Could you check a few things on this model? Use its own coordinates, in mm. Coordinates: 2 decimals unless noted, no trailing zeros. Loops run counter-clockwise (first coordinate to the right, second up) from the corner with the lowest first, then second, coordinate; pieces in that order, holes last. Notation, with made-up numbers: M 62.25,-8.5 L 117.25,-8.5 A22 cw 117.25,7.5 Z; hole C 57.25,-32.75 d1. An arc over 180 degrees is marked long. Write each question's results on one line, items separated by ' | '.
```python
from build123d import *

# Parameters (mm, degrees)
SKETCH2_W           = 31.75
SKETCH2_H           = 22.86
SKETCH2_R           = 3.2766
SKETCH2_H_2         = 12.7
SKETCH2_R_2         = 2.0828
SKETCH2_H_3         = 10.16
BOSS_EXTRUDE1_DEPTH = 1.5875


with BuildPart() as part:
    # Sketch2 → Boss-Extrude1 (new body)
    # profile 1 of 4: a face of its own
    with BuildSketch(Plane.XY):
        with Locations((15.875, 11.43)):
            Rectangle(SKETCH2_W, SKETCH2_H)
        with Locations((15.875, 11.43)):
            Circle(SKETCH2_R, mode=Mode.SUBTRACT)
    # profile 2 of 4: a face of its own
    with BuildSketch(Plane.XY):
        with Locations((15.875, 29.21)):
            Rectangle(SKETCH2_W, SKETCH2_H_2)
        with Locations((9.525, 29.21)):
            Circle(SKETCH2_R_2, mode=Mode.SUBTRACT)
        with Locations((22.225, 29.21)):
            Circle(SKETCH2_R_2, mode=Mode.SUBTRACT)
    # profile 3 of 4: a face of its own
    with BuildSketch(Plane.XY):
        with Locations((15.875, 40.64)):
            Rectangle(SKETCH2_W, SKETCH2_H_3)
    # profile 4 of 4: a face of its own
    with BuildSketch(Plane.XY):
        Polygon((31.75, 53.041010695), (31.75, 45.72), (0, 45.72), align=None)
    extrude(amount=BOSS_EXTRUDE1_DEPTH)


solid = part.part
```
(1) Imagine slicing it at A-A, the plane y = 11.43. List the corners of the cut face in (x, z) for me.
Reported:
outline: M 0,0 L 12.6,0 L 12.6,1.59 L 0,1.59 Z; M 19.15,0 L 31.75,0 L 31.75,1.59 L 19.15,1.59 Z
(2) Imagine slicing it at B-B, the plane z = 1.2. List the corners of the cut face in (x, y) for me (3 decimals).
Reported:
outline: M 0,0 L 31.75,0 L 31.75,53.041 L 0,45.72 Z; hole C 9.525,29.21 d4.166; hole C 15.875,11.43 d6.553; hole C 22.225,29.21 d4.166
(3) If we mould it in two halves opening along Y, with no side actions, what happens to faces 1 (the flat face through (16, 27, 0)), 2 (the cylindrical face through (20.572, 27.943, 0.783)), 3 (the flat face through (16, 0, 1))? For each: released by +Y, released by -Y, zero draft, split by the parting line, or undercut.
Reported:
face 1: zero draft | face 2: undercut | face 3: released by -Y
(4) Please list where these lines run through material, in increasing order: probe 1 along X at (y, z) = (27.5, 1.1); probe 2 along X at (y, z) = (29.5, 0.7); probe 3 along Y at (x, z) = (20.5, 0.15). Write a range as from..to.
Reported:
probe 1: x = 0..8.34, 10.71..21.04, 23.41..31.75 | probe 2: x = 0..7.46, 11.59..20.16, 24.29..31.75 | probe 3: y = 0..28.04, 30.38..50.45
(5) Imagine slicing it at C-C, the plane y = 29.21. List the corners of the cut face in (x, z) for me.
Reported:
outline: M 0,0 L 7.44,0 L 7.44,1.59 L 0,1.59 Z; M 11.61,0 L 20.14,0 L 20.14,1.59 L 11.61,1.59 Z; M 24.31,0 L 31.75,0 L 31.75,1.59 L 24.31,1.59 Z
(6) Will this pin go through, and if not, where does the flat tip stop? P1, Ø3.5, axis at x = 22.225, y = 29.21, coming from the +Z side.
Reported:
P1: passes through
(7) Imagine slicing it at D-D, the plane x = 11. List the corners of the cut face in (y, z) for me.
Reported:
outline: M 0,0 L 27.74,0 L 27.74,1.59 L 0,1.59 Z; M 30.68,0 L 48.26,0 L 48.26,1.59 L 30.68,1.59 Z
